Design review of the part built by this model. Coordinates are the model's own, in mm. Face numbers are marked on the shaded views. Round coordinates to 2 decimals unless told otherwise and drop trailing zeros. Loops run counter-clockwise (first coordinate to the right, second up) from the corner with the lowest first, then second, coordinate; pieces in that order, holes last. Notation, with made-up numbers: (5.5, -17.75) - (28.5, -17.75) arc R20 cw to (28.5, 19.25) - close; hole circle Ø11 at (48.5, 81). An arc over 180 degrees is marked (long way). Answer as CSV lines item,"result". Start each with the question number.
(1) Consider section D-D (z = 16). Give the boundary of the cut face in (x, y) (3 decimals), and give its area (3 significant figures).
(2) Mouldability with a two-part tool opening along X and no side actions: class the marked faces 1, 2 and 3 as released by +X, released by -X, zero draft, split by the parting line, or undercut.
(3) Consider section B-B (y = 0). Give the boundary of the cut face in (x, z) (3 decimals).
(4) For P1, Ø2, axis at x = -15.5, y = 15.5, coming from the +Z side; P2, Ø12, axis at y = -13, z = 18, coming from the -X side; P3, Ø3, axis at x = -47.5, z = 29.5, coming from the -Y side; P4, Ø2, axis at x = -20, y = -45.5, coming from the +Z side, all flat-tipped, find the tip position at first contact; note any pin that passes through.
(5) Consider section A-A (x = 0). Give the boundary of the cut face in (y, z) (3 decimals), and give its area (3 significant figures).
(6) Consider section C-C (z = 24). Give the boundary of the cut face in (x, y) (3 decimals).
(7) Wall thickness on L1, parallel to Y at x = 0, z = 26 (3 decimals); L2, parallel to Z at x = 48.5, y = 22.5; L3, parallel to X at y = 48, z = 14: over which ranges is each line inside the solid? List them lowest first.
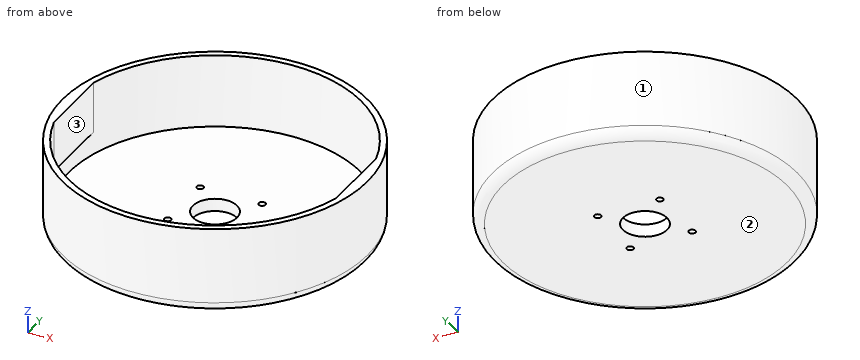
from build123d import *

# Parameters (mm, degrees)
F0_R      = 76.2
F1_DEPTH  = 43.18
F2_R      = 73.025
F3_DEPTH  = 36.83
F4_R      = 11.049
F5_DEPTH  = 25.4
F6_R      = 1.6999966
F7_DEPTH  = 43.181
F8_R      = 5.08
F10_DEPTH = 25.4


with BuildPart() as f1:
    # F0 (on Top) → F1 (new body)
    with BuildSketch(Plane.XY):
        Circle(F0_R)
    extrude(amount=F1_DEPTH)

    # F2 (on face) → F3 (cut)
    with BuildSketch(Plane.XY.offset(43.18)):
        Circle(F2_R)
    extrude(amount=-F3_DEPTH, mode=Mode.SUBTRACT)

    # F4 (on face) → F5 (cut)
    with BuildSketch(Plane(origin=(0, 0, 0), x_dir=(1, 0, 0), z_dir=(0, 0, -1))):
        Circle(F4_R)
    extrude(amount=-F5_DEPTH, mode=Mode.SUBTRACT)

    # F6 (on face) → F7 (cut, through all)
    with BuildSketch(Plane(origin=(0, 0, 0), x_dir=(1, 0, 0), z_dir=(0, 0, -1))):
        with Locations((15.499969, 15.499969)):
            Circle(F6_R)
        with Locations((15.499969, -15.499969)):
            Circle(F6_R)
        with Locations((-15.499969, -15.499969)):
            Circle(F6_R)
        with Locations((-15.499969, 15.499969)):
            Circle(F6_R)
    extrude(amount=-F7_DEPTH, mode=Mode.SUBTRACT)

    # F8
    f8_edges = [f1.edges().sort_by_distance(p)[0] for p in [
        (-76.2, 0, 0),
    ]]
    fillet(f8_edges, radius=F8_R)

    # F9 (on face) → F10 (join)
    with BuildSketch(Plane.XY.offset(43.18)):
        with BuildLine():
            Line((-70.496440513, 0), (-70.496440513, 19.05))
            ThreePointArc((-70.496440513, 19.05), (-73.025, 0), (-70.496440513, -19.05))
            Line((-70.496440513, -19.05), (-70.496440513, 0))
        make_face()
        with BuildLine():
            ThreePointArc((73.025, 0), (72.3901001293, 9.6085393411), (70.496440513, 19.05))
            Line((70.496440513, 19.05), (70.496440513, 0))
            Line((70.496440513, 0), (70.496440513, -19.05))
            ThreePointArc((70.496440513, -19.05), (72.3901001293, -9.6085393411), (73.025, 0))
        make_face()
    extrude(amount=-F10_DEPTH)


solid = f1.part
Determined:
1,outline,"circle Ø152.4 at (0, 0); hole circle Ø146.05 at (0, 0)"
1,area,"1,490 mm^2"
2,face 1,"split by the parting line"
2,face 2,"zero draft"
2,face 3,"undercut"
3,outline,"(-76.2, 5.08) arc R5.08 ccw to (-71.12, 0) - (-11.049, 0) - (-11.049, 6.35) - (-73.025, 6.35) - (-73.025, 17.78) - (-70.496, 17.78) - (-70.496, 43.18) - (-76.2, 43.18) - close; (11.049, 0) - (71.12, 0) arc R5.08 ccw to (76.2, 5.08) - (76.2, 43.18) - (70.496, 43.18) - (70.496, 17.78) - (73.025, 17.78) - (73.025, 6.35) - (11.049, 6.35) - close"
4,P1,"passes through"
4,P2,"stops at x = -75.88"
4,P3,"stops at y = -60.75"
4,P4,"stops at z = 6.35"
5,outline,"(-76.2, 5.08) arc R5.08 ccw to (-71.12, 0) - (-11.049, 0) - (-11.049, 6.35) - (-73.025, 6.35) - (-73.025, 43.18) - (-76.2, 43.18) - close; (11.049, 0) - (71.12, 0) arc R5.08 ccw to (76.2, 5.08) - (76.2, 43.18) - (73.025, 43.18) - (73.025, 6.35) - (11.049, 6.35) - close"
5,area,"1,050 mm^2"
6,outline,"circle Ø152.4 at (0, 0); hole (-70.496, -19.05) arc R73.025 ccw to (70.496, -19.05) - (70.496, 19.05) arc R73.025 ccw to (-70.496, 19.05) - close"
7,L1,"y = -76.2 to -73.025, 73.025 to 76.2"
7,L2,"z = 0 to 6.35"
7,L3,"x = -59.18 to -55.03, 55.03 to 59.18"
